from build123d import *

# Parameters (mm, degrees)
CHAMFER_1_SIZE           = 1
PATTERN_CIRCULAR_2_COUNT = 4


with BuildPart() as part:
    # Эскиз1 → Повернуть1 (revolve)
    with BuildSketch(Plane.XY):
        Polygon((0, 54.75), (60, 54.75), (60, 40), (57, 40), (57, 51.5), (0, 51.5), align=None)
    revolve(axis=Axis((0, 0, 0), (1, 0, 0)))

    # Фаска1
    chamfer_1_edges = [part.edges().sort_by_distance(p)[0] for p in [
        (0, -51.5, 0),
        (57, -40, 0),
        (60, -40, 0),
        (60, -54.75, 0),
        (0, -54.75, 0),
    ]]
    chamfer(chamfer_1_edges, length=CHAMFER_1_SIZE)

    # Эскиз5 → Зенковка для винта с потайной головкой и внутренним шестигранником M31 (revolve, cut)
    with BuildSketch(Plane(origin=(57, 46, 0), x_dir=(0, 0, 1), z_dir=(0, 1, 0))):
        Polygon((0, 0), (0, 22.5), (1.7, 21.478536948), (1.7, 1.77), (3.47, 0), align=None)
    hole_wizard_m31 = revolve(axis=Axis((50.65, 46, 0), (1, 0, 0)), mode=Mode.SUBTRACT)

    # Круговой массив2: Зенковка для винта с потайной головкой и внутренним шестигранником M31 ×4 about axis
    pattern_circular_2_axis = Axis((0, 0, 0), (1, 0, 0))
    for i in range(1, PATTERN_CIRCULAR_2_COUNT):
        add(hole_wizard_m31.rotate(pattern_circular_2_axis, i * 360 / PATTERN_CIRCULAR_2_COUNT), mode=Mode.SUBTRACT)


solid = part.part
Design review of the part built by this model. Coordinates are the model's own, in mm. A direction names the side the tool comes from. Coordinates: 2 decimals unless noted, no trailing zeros. Write each loop counter-clockwise with the first axis right and the second up, starting at its lowest first coordinate (ties: lowest second). Pieces come first, ordered by that corner, then holes. Notation, with made-up numbers: (10.5, 17) - (68.5, 17) arc R25 ccw to (68.5, 31) - close; hole circle Ø6 at (65.5, 7.5). An arc over 180 degrees is marked (long way). One line per item, written item: value.
1) To check wall thickness, follow probe 1 along Z at (x, y) = (59.1, 0); probe 2 along Z at (x, y) = (59, 0); probe 3 along Z at (x, y) = (37, 0). State the ranges of each line that lie inside material, in increasing order.
Answer sheet:
probe 1: z = -54.65 to -47.7, -44.3 to -40.1, 40.1 to 44.3, 47.7 to 54.65
probe 2: z = -54.75 to -47.7, -44.3 to -40, 40 to 44.3, 47.7 to 54.75
probe 3: z = -54.75 to -51.5, 51.5 to 54.75
2) Mouldability with a two-part tool opening along Y and no side actions: class faces 1 (the face through (0, -12, -52)), 2 (the face through (58.659, 0.236, 44.205)), 3 (the face through (30.406, -11.869, -53.448)) as +Y half, -Y half, draft (parallel to the pull), parting line (faces both ways), or undercut.
Answer sheet:
face 1: draft
face 2: undercut
face 3: parting line
3) For faces 4 (the face through (59.38, 0.37, 47.66)), 5 (the face through (57, -23, 35)), list the 3-axis set-ups (+Z, -Z, +X, -X, +Y, -Y) from which the entire face can be reached by the end or side of a thin tool; tool diameter is ignored.
Answer sheet:
face 4: +X, -X
face 5: -X
4) Add section C-C (x = 17). State the section outline as (y, z) points, plus the area to 3 significant figures.
Answer sheet:
outline: circle Ø109.5 at (0, 0); hole circle Ø103 at (0, 0)
area: 1,080 mm2
5) Insertion check: pin 1 (4 mm diameter, centred on x = 40, y = 15, fed in from +Z); pin 2 (2 mm diameter, centred on y = -4.5, z = -44, fed in from -X); pin 3 (4 mm diameter, centred on x = 49.5, z = -40, fed in from +Y); pin 4 (3 mm diameter, centred on y = -46, z = 0, fed in from +X). Each pin has a flat end and moves straight along its axis. Give the tip position at first contact, or say it passes through.
Answer sheet:
pin 1: stops at z = 53.18
pin 2: stops at x = 57
pin 3: stops at y = 39.42
pin 4: passes through
6) Add section A-A (z = 0). Give the number of separate pieces and of enclosed holes in the cut face, plus the area to 3 significant figures.
Answer sheet:
separate pieces: 4
enclosed holes: 0
area: 427 mm2
